from build123d import *

# Parameters (mm, degrees)
SKETCH1_R           = 2.4
BOSS_EXTRUDE1_DEPTH = 7.8
SKETCH2_R           = 3.05
CUT_EXTRUDE1_DEPTH  = 0.8
SKETCH3_R           = 3.05
CUT_EXTRUDE2_DEPTH  = 0.8


with BuildPart() as part:
    # Sketch1 → Boss-Extrude1 (new body)
    with BuildSketch(Plane(origin=(0, 0, 0), x_dir=(1, 0, 0), z_dir=(0, 1, 0))):
        with BuildLine():
            Line((15.06695764, 3.65), (-31.62850949, 3.65))
            ThreePointArc((-31.62850949, 3.65), (-35.27850949, 0), (-31.62850949, -3.65))
            Line((-31.62850949, -3.65), (16.61149051, -3.65))
            ThreePointArc((16.61149051, -3.65), (18.033912451, -3.361430621), (19.23142074, -2.541351135))
            Line((19.23142074, -2.541351135), (35.979469964, 14.72489695))
            Line((35.979469964, 14.72489695), (36.014632418, 14.760846213))
            ThreePointArc((36.014632418, 14.760846213), (36.787004293, 15.9395566), (37.055282295, 17.323010033))
            Line((37.055282295, 17.323010033), (37.055327398, 33.403010033))
            ThreePointArc((37.055327398, 33.403010033), (33.405295822, 37.05304161), (29.755264245, 33.403010033))
            Line((29.755264245, 33.403010033), (29.755264245, 18.792472031))
            Line((29.755264245, 18.792472031), (15.06695764, 3.65))
        make_face()
        Polygon((-30.72850949, 2.4), (-30.72850949, 0.9), (-29.22850949, 0.9), (-29.22850949, -0.9), (-30.72850949, -0.9), (-30.72850949, -2.4), (-32.52850949, -2.4), (-32.52850949, -0.9), (-34.02850949, -0.9), (-34.02850949, 0.9), (-32.52850949, 0.9), (-32.52850949, 2.4), align=None, mode=Mode.SUBTRACT)
        with Locations((-23.58850949, 0)):
            Circle(SKETCH1_R, mode=Mode.SUBTRACT)
        with Locations((-15.54850949, 0)):
            Circle(SKETCH1_R, mode=Mode.SUBTRACT)
        with Locations((-7.50850949, 0)):
            Circle(SKETCH1_R, mode=Mode.SUBTRACT)
        with Locations((0.53149051, 0)):
            Circle(SKETCH1_R, mode=Mode.SUBTRACT)
        with Locations((8.57149051, 0)):
            Circle(SKETCH1_R, mode=Mode.SUBTRACT)
        with Locations((16.61149051, 0)):
            Circle(SKETCH1_R, mode=Mode.SUBTRACT)
        with BuildLine():
            ThreePointArc((23.932119463, 4.099998991), (20.490614709, 4.09600527), (20.583406202, 7.536261171))
            Line((20.583406202, 7.536261171), (26.065029385, 13.19258856))
            ThreePointArc((26.065029385, 13.19258856), (26.083897287, 13.212280453), (26.102987734, 13.231756675))
            ThreePointArc((26.102987734, 13.231756675), (29.48775233, 13.255607669), (29.530054567, 9.871023387))
            Line((29.530054567, 9.871023387), (23.932119463, 4.099998991))
        make_face(mode=Mode.SUBTRACT)
        with Locations((33.405295822, 17.323010033)):
            Circle(SKETCH1_R, mode=Mode.SUBTRACT)
        with Locations((33.405295822, 25.363010033)):
            Circle(SKETCH1_R, mode=Mode.SUBTRACT)
        Polygon((34.305295822, 35.803010033), (34.305295822, 34.303010033), (35.805295822, 34.303010033), (35.805295822, 32.503010033), (34.305295822, 32.503010033), (34.305295822, 31.003010033), (32.505295822, 31.003010033), (32.505295822, 32.503010033), (31.005295822, 32.503010033), (31.005295822, 34.303010033), (32.505295822, 34.303010033), (32.505295822, 35.803010033), align=None, mode=Mode.SUBTRACT)
    extrude(amount=BOSS_EXTRUDE1_DEPTH)

    # Sketch2 → Cut-Extrude1 (cut)
    with BuildSketch(Plane(origin=(0, 7.8, 0), x_dir=(1, 0, 0), z_dir=(0, 1, 0))):
        with Locations((-23.58850949, 0)):
            Circle(SKETCH2_R)
        with Locations((-15.54850949, 0)):
            Circle(SKETCH2_R)
        with Locations((-7.50850949, 0)):
            Circle(SKETCH2_R)
        with Locations((0.53149051, 0)):
            Circle(SKETCH2_R)
        with Locations((8.57149051, 0)):
            Circle(SKETCH2_R)
        with Locations((16.61149051, 0)):
            Circle(SKETCH2_R)
        with Locations((33.405295822, 17.323010033)):
            Circle(SKETCH2_R)
        with Locations((33.405295822, 25.363010033)):
            Circle(SKETCH2_R)
    extrude(amount=-CUT_EXTRUDE1_DEPTH, mode=Mode.SUBTRACT)

    # Sketch3 → Cut-Extrude2 (cut)
    with BuildSketch(Plane.XZ):
        with Locations((-23.55968241, 0)):
            Circle(SKETCH3_R)
        with Locations((-15.54850949, 0)):
            Circle(SKETCH3_R)
        with Locations((-7.50850949, 0)):
            Circle(SKETCH3_R)
        with Locations((0.53149051, 0)):
            Circle(SKETCH3_R)
        with Locations((8.57149051, 0)):
            Circle(SKETCH3_R)
        with Locations((16.61149051, 0)):
            Circle(SKETCH3_R)
        with Locations((33.405295822, -17.323010033)):
            Circle(SKETCH3_R)
        with Locations((33.405295822, -25.363010033)):
            Circle(SKETCH3_R)
    extrude(amount=-CUT_EXTRUDE2_DEPTH, mode=Mode.SUBTRACT)


solid = part.part
Read the model definition and answer for the solid it produces. Units are mm, in the model's axes. A direction names the side the tool comes from. Coordinates: 2 decimals unless noted, no trailing zeros. Loops run counter-clockwise (first coordinate to the right, second up) from the corner with the lowest first, then second, coordinate; pieces in that order, holes last.
Q1. The part is cut by section A-A on x = 23. Write down the section's boundary in (y, z), and give its area (3 significant figures).
Q2. Which of the six approach directions +Z, -Z, +X, -X, +Y, -Y give full straight-line access (tool end or side, diameter ignored) to faces 1 (the face through (-30.729, 4, 2)), 2 (the face through (13.564, 0.394, 0.134)), 3 (the face through (-20.77, 7.41, 1.17)), 4 (the face through (22.514, 3.845, -11.327))?
Q3. The mould has two halves that part along X. Classify faces 5 (the face through (34.305, 4, -32)), 6 (the face through (-32, 4, -2.4)), 7 (the face through (8.8, 7.8, -3.2)), 8 (the face through (27.49, 3.85, -5.97)): +X half, -X half, draft (parallel to the pull), parting line (faces both ways), or undercut.
Q4. Consider probe 1 along X at (y, z) = (5, -33); probe 2 along Z at (x, y) = (-30, 2.75); probe 3 along Z at (x, y) = (31.5, 0.5). Determine where each line is inside the solid, lowest interval first.
Q5. The part is cut by section B-B on y = 1.5. Give the number of separate pieces and of enclosed holes in the cut face, and give its area (3 significant figures).
Q6. Each of these flat-tipped pins is pushed along its axis until it touches: pin 1 Ø5 at (x, z) = (16.5, -0.5) entering from -Y; pin 2 Ø0.5 at (y, z) = (4, 0) entering from +X; pin 3 Ø4 at (y, z) = (2.5, -24.5) entering from -X; pin 4 Ø5 at (x, z) = (0.5, -1.5) entering from +Y. Where does it stop, or does it pass through?
Results below:
1. outline: (0, -11.83) - (7.8, -11.83) - (7.8, -10.03) - (0, -10.03) - close; (0, -3.5) - (7.8, -3.5) - (7.8, -1.34) - (0, -1.34) - close
1. area: 30.9 mm2
2. face 1: +Y, -Y
2. face 2: -Y
2. face 3: +Y
2. face 4: -Z, -X, +Y, -Y
3. face 5: undercut
3. face 6: undercut
3. face 7: draft
3. face 8: +X half
4. probe 1: x = 29.76 to 31.01, 35.81 to 37.06
4. probe 2: z = -3.65 to -0.9, 0.9 to 3.65
4. probe 3: z = -36.52 to -34.3, -32.5 to -27.74, -22.98 to -19.7, -14.94 to -10.11
5. separate pieces: 1
5. enclosed holes: 11
5. area: 457 mm2
6. pin 1: stops at y = 0.8
6. pin 2: stops at x = 21.94
6. pin 3: stops at x = 29.76
6. pin 4: stops at y = 7.8
